```python
from build123d import *

# Parameters (mm, degrees)
PAD_DEPTH = 76.2
FILLET_R  = 0.999998


with BuildPart() as part:
    # Sketch → Pad (new body)
    with BuildSketch(Plane.YZ):
        Polygon((0, 0), (101.6, 0), (101.6, 3.175), (4.53437, 3.175), (35.404021, 87.988668), (78.037116, 14.145981), (91.785269, 22.083481), (90.197769, 24.833112), (79.199247, 18.483112), (34.749247, 95.47277), align=None)
    extrude(amount=PAD_DEPTH)

    # Fillet
    fillet_edges = [part.edges().sort_by_distance(p)[0] for p in [
        (0, 53.067185, 3.175),
        (38.1, 101.6, 3.175),
        (76.2, 101.6, 1.5875),
        (0, 101.6, 1.5875),
        (0, 19.969195, 45.581834),
        (76.2, 19.969195, 45.581834),
        (0, 17.374623, 47.736385),
        (0, 56.720568, 51.067325),
        (0, 56.974247, 56.977941),
        (0, 84.698508, 21.658112),
        (0, 84.911193, 18.114731),
        (0, 90.991519, 23.458297),
        (38.1, 90.197769, 24.833112),
        (38.1, 91.785269, 22.083481),
        (76.2, 90.991519, 23.458297),
        (76.2, 53.067185, 3.175),
        (76.2, 17.374623, 47.736385),
        (76.2, 56.720568, 51.067325),
        (76.2, 56.974247, 56.977941),
        (76.2, 84.698508, 21.658112),
        (76.2, 84.911193, 18.114731),
        (38.1, 78.037116, 14.145981),
    ]]
    fillet(fillet_edges, radius=FILLET_R)


solid = part.part
```
Geometry: final body of the model. Coordinates: model frame, mm. A direction names the side the tool comes from. Round coordinates to 2 decimals unless told otherwise and drop trailing zeros. Order: outer loops, then holes, each group sorted by start corner. A loop starts at its lowest first (then second) coordinate and runs counter-clockwise, first axis right, second up. Notation, with made-up numbers: M -5,-12.75 L 6,-12.75 A22 cw 6,-3.75 Z; hole C 48,11 d2. An arc over 180 degrees is marked long. One line per item, written item: value.
(1) Pull-direction query (Y, two-part tool) for faces 4 (the cylindrical face through (0.3, 17.4, 46.97)), 5 (the cylindrical face through (75.899, 20.048, 46.633)), 6 (the flat face through (38, 53, 3.175)), 7 (the cylindrical face through (0.3, 84.85, 18.41)); classes: pulls with the +Y half, pulls with the -Y half, needs draft (parallel to the pull), parting line crosses it, or undercut.
Result sheet:
face 4: pulls with the -Y half
face 5: undercut
face 6: needs draft
face 7: pulls with the +Y half
(2) Pin query (flat end, axial travel): P1, Ø8, axis at x = 9.5, z = 71.5, coming from the +Y side. Return the tip coordinate at first contact, or that it passes through.
Result sheet:
P1: y = 50.9
(3) Cut plane B-B (x = 67.5). Return the cut outline in (y, z) (1 decimal).
Result sheet:
outline: M 0,0 L 101.6,0 L 101.6,2.2 A1 ccw 100.6,3.2 L 4.5,3.2 L 35.4,88 L 77.5,15 A1 ccw 78.9,14.6 L 90.9,21.6 A1 ccw 91.3,22.9 L 90.7,24 A1 ccw 89.3,24.3 L 79.2,18.5 L 34.7,95.5 Z
(4) Reachability of faces 1 (the flat face through (37.581, 19.753, 44.988)), 2 (the cylindrical face through (75.9, 84.85, 18.41)), 3 (the flat face through (37.58, 84.34, 21.45)) from +Z, -Z, +X, -X, +Y, -Y: full face, straight path, thin tool, end or side. Return the list, or none.
Result sheet:
face 1: +X, -X
face 2: +X, +Y
face 3: +Z, +X, -X
(5) Line query: probe 1 along Y at (x, z) = (12, 19); probe 2 along Y at (x, z) = (53, 21); probe 3 along Z at (x, y) = (59.5, 42.5) (3 decimals). Output: solid intervals per line, ascending. Write a range as [from, to].
Result sheet:
probe 1: [6.92, 10.29], [75.23, 78.9], [80.09, 86.44]
probe 2: [7.64, 11.02], [74.08, 77.75], [83.56, 89.91]
probe 3: [0, 3.175], [75.698, 82.048]
(6) Cut plane A-A (y = 94). Return the cut outline in (x, z) (3 decimals).
Result sheet:
outline: M 0,0 L 76.2,0 L 76.2,2.175 A1 ccw 75.2,3.175 L 1,3.175 A1 ccw 0,2.175 Z
